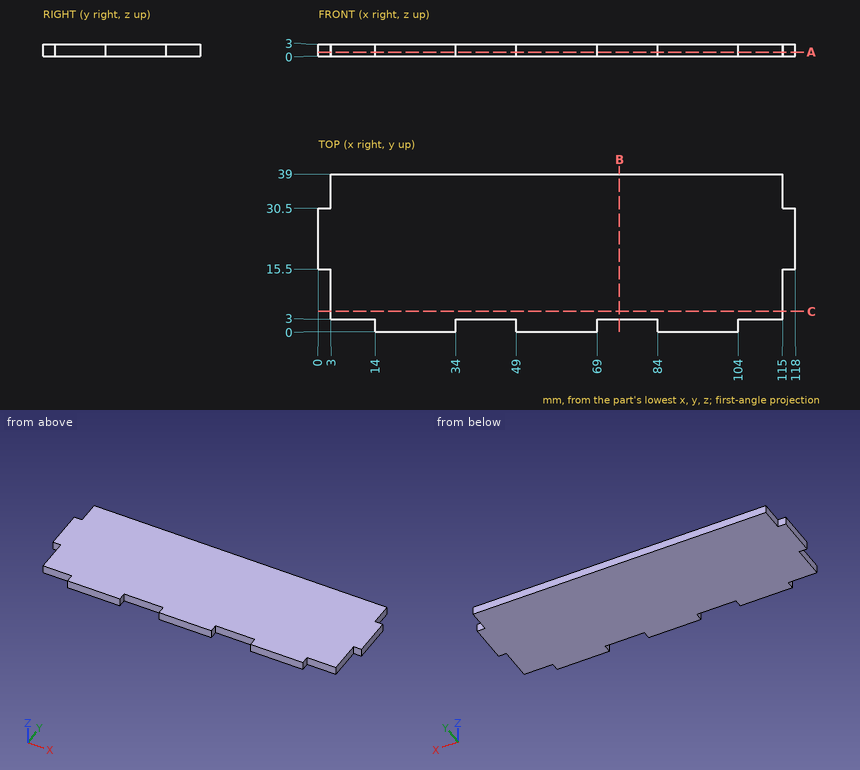
Study the drawing (mm; zero at the part's minimum x, y, z) and answer. Round coordinates to 2 decimals unless told otherwise and drop trailing zeros. Write each loop counter-clockwise with the first axis right and the second up, starting at its lowest first coordinate (ties: lowest second). Pieces come first, ordered by that corner, then holes.
Q1. Find section B-B on x = 74.5. Determine the outline of the cut face in (y, z).
Values:
outline: (3, 0) - (39, 0) - (39, 3) - (3, 3) - close
Q2. Flat-ended cylindrical pins translate along their axes: P1, Ø1.5, axis at y = 10.5, z = 2, coming from the -X side; P2, Ø1.5, axis at x = 78.5, z = 2, coming from the -Y side; P3, Ø0.9, axis at y = 2, z = 1, coming from the -X side; P4, Ø8, axis at x = 95, y = 20.5, coming from the -Z side. Find the tip coordinate at first contact, or state that the pin passes through.
Values:
P1: stops at x = 3
P2: stops at y = 3
P3: stops at x = 14
P4: stops at z = 0
Q3. Find section A-A on z = 1. Determine the outline of the cut face in (x, y), and give its area (3 significant figures).
Values:
outline: (0, 15.5) - (3, 15.5) - (3, 3) - (14, 3) - (14, 0) - (34, 0) - (34, 3) - (49, 3) - (49, 0) - (69, 0) - (69, 3) - (84, 3) - (84, 0) - (104, 0) - (104, 3) - (115, 3) - (115, 15.5) - (118, 15.5) - (118, 30.5) - (115, 30.5) - (115, 39) - (3, 39) - (3, 30.5) - (0, 30.5) - close
area: 4,300 mm2
Q4. Straight lines are drawn through the part: line 1 (Y direction, x = 80, z = 0.75); line 2 (X direction, y = 7.5, z = 0.75). For each, find the intervals that lie inside material, in ascending order.
Values:
line 1: y = 3 to 39
line 2: x = 3 to 115
Q5. Find section C-C on y = 5. Determine the outline of the cut face in (x, z).
Values:
outline: (3, 0) - (115, 0) - (115, 3) - (3, 3) - close
